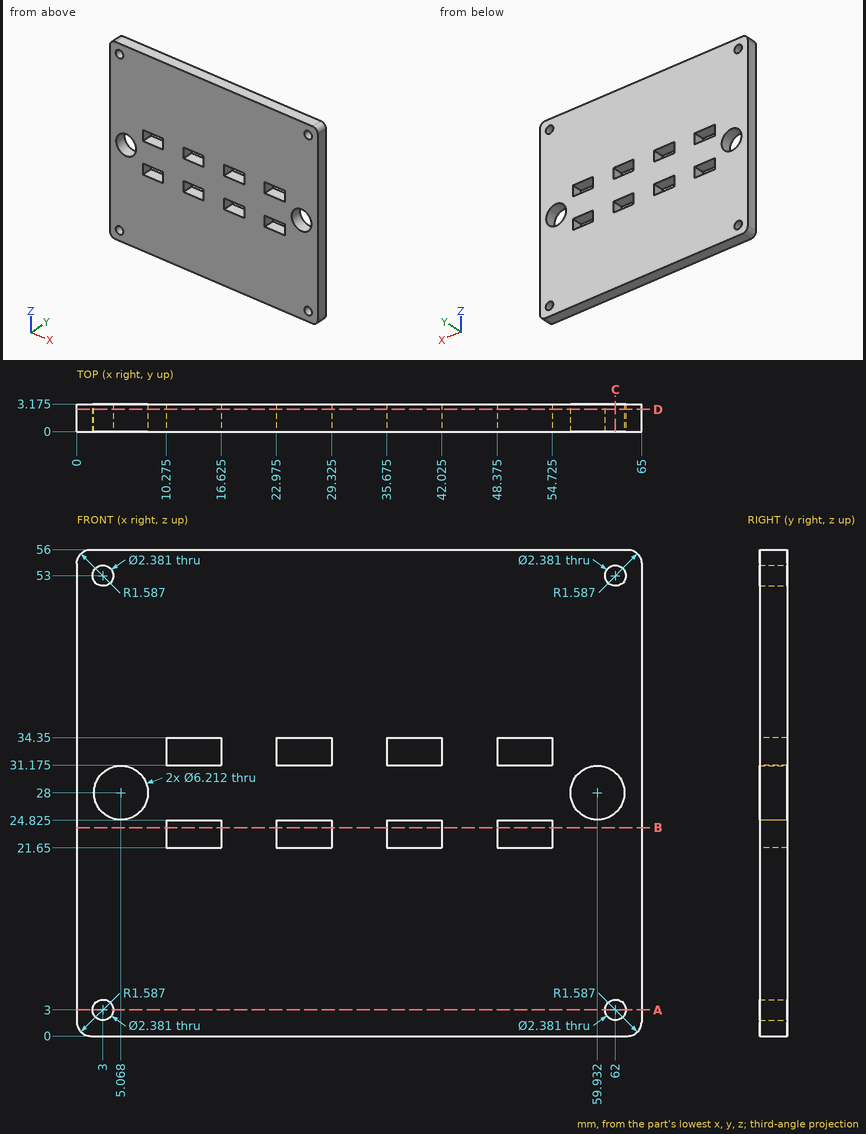
Drawing for the job (mm, zero at the part's lowest x, y, z). Give positions to 0.01 mm unless a question says otherwise; leave off trailing zeros. Order: outer loops, then holes, each group sorted by start corner. A loop starts at its lowest first (then second) coordinate and runs counter-clockwise, first axis right, second up. Notation, with made-up numbers: (-24.5, -5.5) - (27.5, -5.5) arc R27 cw to (27.5, 31.5) - close; hole circle Ø4 at (48.25, 82). An arc over 180 degrees is marked (long way). Use one line per item in the form item = value.
Item 1: Slice it at A-A on z = 3. Give the cut face in (x, y) (1 decimal).
Solution:
outline = (0, 0) - (1.8, 0) - (1.8, 3.2) - (0, 3.2) - close; (4.2, 0) - (60.8, 0) - (60.8, 3.2) - (4.2, 3.2) - close; (63.2, 0) - (65, 0) - (65, 3.2) - (63.2, 3.2) - close
Item 2: Slice it at D-D on y = 2.55. Count the separate pieces of the cut face and the enclosed holes in it, and give its area (3 significant figures).
Solution:
separate_pieces = 1
enclosed_holes = 14
area = 3,400 mm2
Item 3: Pin check, flat tip, straight feed: pin 1 Ø1.4 at (x, z) = (62, 3) entering from -Y. Stop position of the tip, or through.
Solution:
pin_1 = through
Item 4: Slice it at B-B on z = 24. Give the cut face in (x, y) (1 decimal), and give its area (3 significant figures).
Solution:
outline = (0, 0) - (10.3, 0) - (10.3, 3.2) - (0, 3.2) - close; (16.6, 0) - (23, 0) - (23, 3.2) - (16.6, 3.2) - close; (29.3, 0) - (35.7, 0) - (35.7, 3.2) - (29.3, 3.2) - close; (42, 0) - (48.4, 0) - (48.4, 3.2) - (42, 3.2) - close; (54.7, 0) - (65, 0) - (65, 3.2) - (54.7, 3.2) - close
area = 126 mm2
Item 5: Slice it at C-C on x = 62. Give the cut face in (y, z) (1 decimal).
Solution:
outline = (0, 0) - (3.2, 0) - (3.2, 1.8) - (0, 1.8) - close; (0, 4.2) - (3.2, 4.2) - (3.2, 25.7) - (0, 25.7) - close; (0, 30.3) - (3.2, 30.3) - (3.2, 51.8) - (0, 51.8) - close; (0, 54.2) - (3.2, 54.2) - (3.2, 56) - (0, 56) - close
Item 6: Probe probe 1 along X at (y, z) = (1.65, 3); probe 2 along X at (y, z) = (0.7, 34) (1 decimal); probe 3 along Z at (x, y) = (3.5, 0.75). List the from-to ranges inside material, lowest first. Write a range as from..to.
Solution:
probe_1 = 0..1.81, 4.19..60.81, 63.19..65
probe_2 = 0..10.3, 16.6..23, 29.3..35.7, 42..48.4, 54.7..65
probe_3 = 0..1.92, 4.08..25.32, 30.68..51.92, 54.08..56
